from build123d import *

# Parameters (mm, degrees)
ESBO_O1_W             = 39
ESBO_O1_H             = 70
FLANGE_BASE1_DEPTH    = 20
ESBO_O6_R             = 2.1
CORTE_EXTRUS_O1_DEPTH = 15
ESBO_O8_R             = 4.25
CORTE_EXTRUS_O2_DEPTH = 39


# Sheet-metal steps are written as plain solids
with BuildPart() as part:
    # Esboço1 → Flange-base1 (new body)
    with BuildSketch(Plane(origin=(0, 0, 0), x_dir=(1, 0, 0), z_dir=(0, 1, 0))):
        Rectangle(ESBO_O1_W, ESBO_O1_H)
    extrude(amount=-FLANGE_BASE1_DEPTH)

    # Esboço6 → Corte-extrusão1 (cut)
    with BuildSketch(Plane(origin=(0, 0, 0), x_dir=(1, 0, 0), z_dir=(0, 1, 0))):
        with Locations(Location((-15, 12, 0), (0, 0, 270))):
            Circle(ESBO_O6_R)
        with Locations(Location((15, 12, 0), (0, 0, 270))):
            Circle(ESBO_O6_R)
        with Locations(Location((0, 12, 0), (0, 0, 270))):
            Circle(ESBO_O6_R)
        with Locations(Location((-15, -12, 0), (0, 0, 270))):
            Circle(ESBO_O6_R)
        with Locations(Location((0, -12, 0), (0, 0, 270))):
            Circle(ESBO_O6_R)
        with Locations(Location((15, -12, 0), (0, 0, 270))):
            Circle(ESBO_O6_R)
    extrude(amount=-CORTE_EXTRUS_O1_DEPTH, mode=Mode.SUBTRACT)

    # Esboço8 → Corte-extrusão2 (cut)
    with BuildSketch(Plane.ZY.offset(19.5)):
        with Locations((-26, -10.5)):
            Circle(ESBO_O8_R)
        with Locations((26, -10.5)):
            Circle(ESBO_O8_R)
        with Locations((0, -10.5)):
            Circle(ESBO_O8_R)
    extrude(amount=-CORTE_EXTRUS_O2_DEPTH, mode=Mode.SUBTRACT)


solid = part.part
Build history of the part. All positions in model axes, mm. A direction names the side the tool comes from. Round coordinates to 2 decimals unless told otherwise and drop trailing zeros. Order: outer loops, then holes, each group sorted by start corner. A loop starts at its lowest first (then second) coordinate and runs counter-clockwise, first axis right, second up. Notation, with made-up numbers: M 2,19 L 34,19 A25 cw 34,49 Z; hole C 14.25,-39 d8. An arc over 180 degrees is marked long. Use CSV: the item, a comma, the result in double quotes. Start each with the question number.
(1) Drill centre lines: probe 1 along X at (y, z) = (-4, 12); probe 2 along Y at (x, z) = (-7, 0); probe 3 along Z at (x, y) = (9, -8.5). Where is each one in solid material? Low to high.
(2) Cut at A-A on y = -10.5. State how many separate pieces and enclosed holes the cut face has, then the cut area to 3 significant figures.
(3) Cut at B-B on z = 0. List the corners of the cut face in (x, y).
(4) Cut at C-C on x = 6. List the corners of the cut face in (y, z).
(5) Flat gauge pins, fed straight in: P1, Ø1.3, axis at x = 14, z = 12, coming from the +Y side; P2, Ø3.5, axis at x = 15.5, z = -11.5, coming from the +Y side; P3, Ø7.5, axis at y = -10.5, z = -26, coming from the -X side. Where does each tip first touch, or does it go through?
(6) Mould opens along Y. For faces 3 (the face through (-0.27, -13.09, 22.63)), 4 (the face through (-12.918, -7.395, -12.273)), 5 (the face through (-15, -15, 12)), 6 (the face through (-0.27, -13.09, -29.37)) say: +Y half, -Y half, draft (parallel to the pull), parting line (faces both ways), or undercut.
(7) Cut at D-D on z = 12. List the corners of the cut face in (x, y).
(8) Tool access for faces 1 (the face through (15, -15, -12)), 2 (the face through (0, 0, 0)): list every direction of +Z, -Z, +X, -X, +Y, -Y with a clear straight run to the whole face (end or side of a thin tool).
Findings:
1,probe 1,"x = -19.5 to -17.1, -12.9 to -2.1, 2.1 to 12.9, 17.1 to 19.5"
1,probe 2,"y = -20 to -14.75, -6.25 to 0"
1,probe 3,"z = -35 to -29.75, -22.25 to -3.75, 3.75 to 22.25, 29.75 to 35"
2,separate pieces,"4"
2,enclosed holes,"6"
2,area,"1,650 mm^2"
3,outline,"M -19.5,-20 L 19.5,-20 L 19.5,-14.75 L -19.5,-14.75 Z; M -19.5,-6.25 L 19.5,-6.25 L 19.5,0 L -19.5,0 Z"
4,outline,"M -20,-35 L 0,-35 L 0,35 L -20,35 Z; hole C -10.5,-26 d8.5; hole C -10.5,0 d8.5; hole C -10.5,26 d8.5"
5,P1,"stops at y = -15"
5,P2,"stops at y = 0"
5,P3,"passes through"
6,face 3,"undercut"
6,face 4,"draft"
6,face 5,"+Y half"
6,face 6,"undercut"
7,outline,"M -19.5,-20 L 19.5,-20 L 19.5,0 L 17.1,0 L 17.1,-15 L 12.9,-15 L 12.9,0 L 2.1,0 L 2.1,-15 L -2.1,-15 L -2.1,0 L -12.9,0 L -12.9,-15 L -17.1,-15 L -17.1,0 L -19.5,0 Z"
8,face 1,"+Y"
8,face 2,"+Z, -Z, +X, -X, +Y"
